Build history of the part. All positions in model axes, mm. A direction names the side the tool comes from. Give positions to 0.01 mm unless a question says otherwise; leave off trailing zeros. Loops run counter-clockwise (first coordinate to the right, second up) from the corner with the lowest first, then second, coordinate; pieces in that order, holes last. Notation, with made-up numbers: M 33.25,10 L 85.25,10 A20 ccw 85.25,49 Z; hole C -36,-16.5 d3. An arc over 180 degrees is marked long. Answer as a JSON object with one key per item and string values. Group by question number.
1. Drill centre lines: line 1 along Y through (x, z) = (-36.5, 4.5); line 2 along Y through (x, z) = (0, 4); line 3 along Y through (x, z) = (-36.5, 1.65). Where is each one in solid material? Low to high. Write a range as [from, to].
2. Slice it at D-D (x = 2). List the corners of the cut face in (y, z), then the cut area to 3 significant figures.
3. 3-axis set-ups, long thin cutter, end or side, ignore diameter. For faces 1 (the face through (-1, -75, 3)), 2 (the face through (-34.19, 70.54, 4.54)), 3 (the face through (-33, 33, 3)), 4 (the face through (-5, -60, 3)): which of +Z, -Z, +X, -X, +Y, -Y reach the whole face in a straight line?
4. Slice it at A-A (x = -13). List the corners of the cut face in (y, z), then the cut area to 3 significant figures.
5. Slice it at C-C (x = -30.5). List the corners of the cut face in (y, z), then the cut area to 4 significant figures.
6. Slice it at B-B (y = 62). List the corners of the cut face in (x, z), then the cut area to 3 significant figures.
7. Drop flat-ended pins along their axis: pin 1 Ø3 at (x, y) = (36.5, 71.5) entering from +Z; pin 2 Ø1.6 at (x, y) = (36.5, -71.5) entering from -Z; pin 3 Ø5.5 at (x, y) = (-13, -42) entering from +Z. Give the stop position or say it passes through.
from build123d import *

# Parameters (mm, degrees)
SKETCH1_W           = 80
SKETCH1_H           = 150
SKETCH1_W_2         = 66
SKETCH1_H_2         = 136
BOSS_EXTRUDE1_DEPTH = 7
SKETCH2_W           = 66
SKETCH2_H           = 36
BOSS_EXTRUDE2_DEPTH = 7
SKETCH3_R           = 5.5
CUT_EXTRUDE1_DEPTH  = 86.287748241
SKETCH4_R           = 6.05
CUT_EXTRUDE2_DEPTH  = 5.6
SKETCH5_R           = 11
CUT_EXTRUDE3_DEPTH  = 3
SKETCH6_R           = 1.6
CUT_EXTRUDE4_DEPTH  = 86.287748241
SKETCH7_W           = 50
SKETCH7_H           = 38
CUT_EXTRUDE5_DEPTH  = 1
SKETCH8_R           = 3
CUT_EXTRUDE6_DEPTH  = 3
SKETCH9_R           = 1.35
CUT_EXTRUDE7_DEPTH  = 86.287748241
SKETCH10_R          = 2.5
CUT_EXTRUDE8_DEPTH  = 5
CHAMFER1_SIZE       = 2
SKETCH11_W          = 66
SKETCH11_H          = 30.5
BOSS_EXTRUDE3_DEPTH = 7
SKETCH12_R          = 1.35
CUT_EXTRUDE9_DEPTH  = 86.287748241
SKETCH13_R          = 2.5
CUT_EXTRUDE10_DEPTH = 5


with BuildPart() as part:
    # Sketch1 → Boss-Extrude1 (new body)
    with BuildSketch(Plane.XY):
        Rectangle(SKETCH1_W, SKETCH1_H)
        Rectangle(SKETCH1_W_2, SKETCH1_H_2, mode=Mode.SUBTRACT)
    extrude(amount=BOSS_EXTRUDE1_DEPTH)

    # Sketch2 → Boss-Extrude2 (add)
    with BuildSketch(Plane.XY.offset(7)):
        with Locations((0, -50)):
            Rectangle(SKETCH2_W, SKETCH2_H)
    extrude(amount=-BOSS_EXTRUDE2_DEPTH)

    # Sketch3 → Cut-Extrude1 (cut, through all)
    with BuildSketch(Plane(origin=(0, 0, 0), x_dir=(-1, 0, 0), z_dir=(0, 0, -1))):
        with Locations((0, -55)):
            Circle(SKETCH3_R)
    extrude(amount=-CUT_EXTRUDE1_DEPTH, mode=Mode.SUBTRACT)

    # Sketch4 → Cut-Extrude2 (cut)
    with BuildSketch(Plane(origin=(0, 0, 0), x_dir=(-1, 0, 0), z_dir=(0, 0, -1))):
        with Locations((0, -55)):
            Circle(SKETCH4_R)
    extrude(amount=-CUT_EXTRUDE2_DEPTH, mode=Mode.SUBTRACT)

    # Sketch5 → Cut-Extrude3 (cut)
    with BuildSketch(Plane(origin=(0, 0, 0), x_dir=(-1, 0, 0), z_dir=(0, 0, -1))):
        with Locations((0, -55)):
            Circle(SKETCH5_R)
    extrude(amount=-CUT_EXTRUDE3_DEPTH, mode=Mode.SUBTRACT)

    # Sketch6 → Cut-Extrude4 (cut, through all)
    with BuildSketch(Plane(origin=(0, 0, 0), x_dir=(-1, 0, 0), z_dir=(0, 0, -1))):
        with Locations((-13, -42)):
            Circle(SKETCH6_R)
        with Locations((13, -42)):
            Circle(SKETCH6_R)
        with Locations((13, -68)):
            Circle(SKETCH6_R)
        with Locations((-13, -68)):
            Circle(SKETCH6_R)
    extrude(amount=-CUT_EXTRUDE4_DEPTH, mode=Mode.SUBTRACT)

    # Sketch7 → Cut-Extrude5 (cut)
    with BuildSketch(Plane(origin=(0, 0, 0), x_dir=(-1, 0, 0), z_dir=(0, 0, -1))):
        with Locations((0, -55)):
            Rectangle(SKETCH7_W, SKETCH7_H)
    extrude(amount=-CUT_EXTRUDE5_DEPTH, mode=Mode.SUBTRACT)

    # Sketch8 → Cut-Extrude6 (cut)
    with BuildSketch(Plane.XY.offset(7)):
        with Locations((-13, -42)):
            Circle(SKETCH8_R)
        with Locations((13, -42)):
            Circle(SKETCH8_R)
        with Locations((13, -68)):
            Circle(SKETCH8_R)
        with Locations((-13, -68)):
            Circle(SKETCH8_R)
    extrude(amount=-CUT_EXTRUDE6_DEPTH, mode=Mode.SUBTRACT)

    # Sketch9 → Cut-Extrude7 (cut, through all)
    with BuildSketch(Plane.XY.offset(7)):
        with Locations((-36.5, 71.5)):
            Circle(SKETCH9_R)
        with Locations((36.5, 71.5)):
            Circle(SKETCH9_R)
        with Locations((-36.5, -71.5)):
            Circle(SKETCH9_R)
        with Locations((36.5, -71.5)):
            Circle(SKETCH9_R)
        with Locations((-36.5, 35.5)):
            Circle(SKETCH9_R)
        with Locations((36.5, 35.5)):
            Circle(SKETCH9_R)
        with Locations((36.5, -26.5)):
            Circle(SKETCH9_R)
        with Locations((-36.5, -26.5)):
            Circle(SKETCH9_R)
    extrude(amount=-CUT_EXTRUDE7_DEPTH, mode=Mode.SUBTRACT)

    # Sketch10 → Cut-Extrude8 (cut)
    with BuildSketch(Plane.XY.offset(7)):
        with Locations((-36.5, 71.5)):
            Circle(SKETCH10_R)
        with Locations((36.5, 35.5)):
            Circle(SKETCH10_R)
        with Locations((-36.5, 35.5)):
            Circle(SKETCH10_R)
        with Locations((36.5, 71.5)):
            Circle(SKETCH10_R)
        with Locations((-36.5, -71.5)):
            Circle(SKETCH10_R)
        with Locations((36.5, -71.5)):
            Circle(SKETCH10_R)
        with Locations((-36.5, -26.5)):
            Circle(SKETCH10_R)
        with Locations((36.5, -26.5)):
            Circle(SKETCH10_R)
    extrude(amount=-CUT_EXTRUDE8_DEPTH, mode=Mode.SUBTRACT)

    # Chamfer1
    # the kernel refuses this chamfer: 2 mm, written as the material it takes off along each edge
    with BuildSketch(Plane(origin=(-40, 80.143365976, 7), x_dir=(-0.027495876610585623, 0, -0.9996219169112968), z_dir=(0, -1, 0)), Plane(origin=(40, -80.143365976, 7), x_dir=(0.027495876610585623, 0, -0.9996219169112968), z_dir=(0, 1, 0))) as chamfer1_piece_1:
        Polygon((CHAMFER1_SIZE * 0.999621916911, CHAMFER1_SIZE * 0.0274958766106), (-CHAMFER1_SIZE * 0.0274958766106, CHAMFER1_SIZE * 0.999621916911), (0, 0), align=None)
    extrude(amount=160.286731952, mode=Mode.SUBTRACT)

    # Sketch11 → Boss-Extrude3 (add)
    with BuildSketch(Plane.XY.offset(7)):
        with Locations((0, -16.75)):
            Rectangle(SKETCH11_W, SKETCH11_H)
    extrude(amount=-BOSS_EXTRUDE3_DEPTH)

    # Sketch12 → Cut-Extrude9 (cut, through all)
    with BuildSketch(Plane.XY.offset(7)):
        with Locations((-20, 71.5)):
            Circle(SKETCH12_R)
        with Locations((20, 71.5)):
            Circle(SKETCH12_R)
    extrude(amount=-CUT_EXTRUDE9_DEPTH, mode=Mode.SUBTRACT)

    # Sketch13 → Cut-Extrude10 (cut)
    with BuildSketch(Plane.XY.offset(7)):
        with Locations((-20, 71.5)):
            Circle(SKETCH13_R)
        with Locations((20, 71.5)):
            Circle(SKETCH13_R)
    extrude(amount=-CUT_EXTRUDE10_DEPTH, mode=Mode.SUBTRACT)


solid = part.part
Established:
{
 "1": {"line 1": "y = [-75, -74], [-69, -29], [-24, 33], [38, 69], [74, 75]", "line 2": "y = [-75, -61.05], [-48.95, -1.5], [68, 75]", "line 3": "y = [-75, -72.85], [-70.15, -27.85], [-25.15, 34.15], [36.85, 70.15], [72.85, 75]"},
 "2": {"outline": "M -75,0 L -74,0 L -74,1 L -65.82,1 L -65.82,3 L -60.71,3 L -60.71,5.6 L -60.12,5.6 L -60.12,7 L -75,7 Z; M -49.88,5.6 L -49.29,5.6 L -49.29,3 L -44.18,3 L -44.18,1 L -36,1 L -36,0 L -1.5,0 L -1.5,7 L -49.88,7 Z; M 68,0 L 75,0 L 75,7 L 68,7 Z", "area": "438 mm^2"},
 "3": {"face 1": "+Z, -Z, +X, -X, -Y", "face 2": "+Z", "face 3": "+Z, -Z", "face 4": "-Z"},
 "4": {"outline": "M -75,0 L -74,0 L -74,1 L -69.6,1 L -69.6,4 L -71,4 L -71,7 L -75,7 Z; M -66.4,1 L -43.6,1 L -43.6,4 L -45,4 L -45,7 L -65,7 L -65,4 L -66.4,4 Z; M -40.4,1 L -36,1 L -36,0 L -1.5,0 L -1.5,7 L -39,7 L -39,4 L -40.4,4 Z; M 68,0 L 75,0 L 75,7 L 68,7 Z", "area": "470 mm^2"},
 "5": {"outline": "M -75,0 L -1.5,0 L -1.5,7 L -75,7 Z; M 68,0 L 75,0 L 75,7 L 68,7 Z", "area": "563.5 mm^2"},
 "6": {"outline": "M -40,0 L -33,0 L -33,7 L -38,7 L -40,5 Z; M 33,0 L 40,0 L 40,5 L 38,7 L 33,7 Z", "area": "94.0 mm^2"},
 "7": {"pin 1": "stops at z = 2", "pin 2": "passes through", "pin 3": "stops at z = 4"}
}
